Read the model definition and answer for the solid it produces. Units are mm, in the model's axes. A direction names the side the tool comes from. Coordinates: 2 decimals unless noted, no trailing zeros. Loops run counter-clockwise (first coordinate to the right, second up) from the corner with the lowest first, then second, coordinate; pieces in that order, holes last. Notation, with made-up numbers: (75, 17.5) -> (85, 17.5) arc R20 ccw to (85, 46.5) -> close; hole circle Ø5 at (-13.5, -26). An arc over 180 degrees is marked (long way). Answer as a JSON object with one key per item and string values. Group by question number.
1) Section C-C, the plane x = -3.5 is taken. Give the vertices of the cut face in (y, z), plus the area to 3 significant figures.
2) Section D-D, the plane y = -82.5 is taken. Give the vertices of the cut face in (x, z), plus the area to 3 significant figures.
3) Section B-B, the plane z = 4.4 is taken. Count the separate pieces of the cut face and the enclosed holes in it, plus the area to 3 significant figures.
4) A flat-ended cylindrical pin translates along its axis: P1, Ø3, axis at x = -23.5, z = 3.5, coming from the -Y side. Find the tip coordinate at first contact, or state that the pin passes through.
5) Consider probe 1 along Y at (x, z) = (-23.75, 2); probe 2 along X at (y, z) = (-16, 0.45); probe 3 along Y at (x, z) = (23.75, 1.7). Determine where each line is inside the solid, lowest interval first. Write a range as [from, to].
6) Section A-A, the plane y = 2.58 is taken. Give the vertices of the cut face in (x, z).
7) Determine the mould class of faces 1 (the face through (-49.907, 6.677, 2.839)), 2 (the face through (-6, 12.5, 3)), 3 (the face through (-53.41, -49.93, 2.76)) for opening direction X: released by +X, released by -X, zero draft, split by the parting line, or undercut.
8) Which of the six approach directions +Z, -Z, +X, -X, +Y, -Y give full straight-line access (tool end or side, diameter ignored) to faces 4 (the face through (-20, -3, 3)), 5 (the face through (-63.37, -66.79, 2.84)), 6 (the face through (-23, -12.5, 3))?
from build123d import *

# Parameters (mm, degrees)
BOSS_EXTRU_1_DEPTH      = 5.6
ENL_V_MAT_EXTRU_1_REACH = 135.059
ESQUISSE2_W             = 40
ESQUISSE2_H             = 20
ENL_V_MAT_EXTRU_2_REACH = 135.059
ESQUISSE3_R             = 1.45
CONG_2_R                = 12.5
CONG_3_R                = 10
CONG_4_R                = 30
CONG_5_R                = 30
ENL_V_MAT_EXTRU_3_REACH = 135.059
CONG_6_R                = 2
ENL_V_MAT_EXTRU_4_REACH = 135.059
ESQUISSE5_R             = 1.15


# Some blends are built 0.0001 mm under size
with BuildPart() as part:
    # Esquisse1 → Boss.-Extru.1 (new body)
    with BuildSketch(Plane.XY):
        with BuildLine():
            Line((-32.5, 12.5), (-52.5, 12.5))
            ThreePointArc((-52.5, 12.5), (-69.287355537, -46.339080558), (-67.5, -107.5))
            ThreePointArc((-67.5, -107.5), (-62.5, -112.5), (-57.5, -107.5))
            ThreePointArc((-57.5, -107.5), (-48.914858734, -58.969774017), (-32.5, -12.5))
            Line((-32.5, -12.5), (32.5, -12.5))
            Line((32.5, -12.5), (32.5, 12.5))
            Line((32.5, 12.5), (-32.5, 12.5))
        make_face()
    extrude(amount=BOSS_EXTRU_1_DEPTH)

    # Esquisse2 → Enlèv. mat.-Extru.1 (cut, up to next)
    with BuildSketch(Plane.XY.offset(5.6), mode=Mode.PRIVATE) as enl_v_mat_extru_1_sk1:
        with Locations((0, -2.5)):
            Rectangle(ESQUISSE2_W, ESQUISSE2_H)
    enl_v_mat_extru_1_tool1 = extrude(enl_v_mat_extru_1_sk1.sketch, amount=-ENL_V_MAT_EXTRU_1_REACH, mode=Mode.PRIVATE) & part.part
    add(enl_v_mat_extru_1_tool1.solids().sort_by_distance((0, -2.5, 5.6))[0], mode=Mode.SUBTRACT)

    # Esquisse3 → Enlèv. mat.-Extru.2 (cut, up to next)
    with BuildSketch(Plane.XY.offset(5.6), mode=Mode.PRIVATE) as enl_v_mat_extru_2_sk1:
        with Locations((-23.75, -7.58)):
            Circle(ESQUISSE3_R)
    enl_v_mat_extru_2_tool1 = extrude(enl_v_mat_extru_2_sk1.sketch, amount=-ENL_V_MAT_EXTRU_2_REACH, mode=Mode.PRIVATE) & part.part
    # Esquisse3 → Enlèv. mat.-Extru.2 (cut, up to next)
    with BuildSketch(Plane.XY.offset(5.6), mode=Mode.PRIVATE) as enl_v_mat_extru_2_sk2:
        with Locations((23.75, -7.58)):
            Circle(ESQUISSE3_R)
    enl_v_mat_extru_2_tool2 = extrude(enl_v_mat_extru_2_sk2.sketch, amount=-ENL_V_MAT_EXTRU_2_REACH, mode=Mode.PRIVATE) & part.part
    # Esquisse3 → Enlèv. mat.-Extru.2 (cut, up to next)
    with BuildSketch(Plane.XY.offset(5.6), mode=Mode.PRIVATE) as enl_v_mat_extru_2_sk3:
        with Locations((23.75, 2.58)):
            Circle(ESQUISSE3_R)
    enl_v_mat_extru_2_tool3 = extrude(enl_v_mat_extru_2_sk3.sketch, amount=-ENL_V_MAT_EXTRU_2_REACH, mode=Mode.PRIVATE) & part.part
    # Esquisse3 → Enlèv. mat.-Extru.2 (cut, up to next)
    with BuildSketch(Plane.XY.offset(5.6), mode=Mode.PRIVATE) as enl_v_mat_extru_2_sk4:
        with Locations((-23.75, 2.58)):
            Circle(ESQUISSE3_R)
    enl_v_mat_extru_2_tool4 = extrude(enl_v_mat_extru_2_sk4.sketch, amount=-ENL_V_MAT_EXTRU_2_REACH, mode=Mode.PRIVATE) & part.part
    add(enl_v_mat_extru_2_tool1.solids().sort_by_distance((-23.75, -7.58, 5.6))[0], mode=Mode.SUBTRACT)
    add(enl_v_mat_extru_2_tool2.solids().sort_by_distance((23.75, -7.58, 5.6))[0], mode=Mode.SUBTRACT)
    add(enl_v_mat_extru_2_tool3.solids().sort_by_distance((23.75, 2.58, 5.6))[0], mode=Mode.SUBTRACT)
    add(enl_v_mat_extru_2_tool4.solids().sort_by_distance((-23.75, 2.58, 5.6))[0], mode=Mode.SUBTRACT)

    # Congé2
    cong_2_edges = [part.edges().sort_by_distance(p)[0] for p in [
        (32.5, -12.5, 2.8),
        (32.5, 12.5, 2.8),
    ]]
    fillet(cong_2_edges, radius=CONG_2_R - 0.0001)  # a hair under: the kernel refuses the full size

    # Congé3
    cong_3_edges = [part.edges().sort_by_distance(p)[0] for p in [
        (-32.5, -12.5, 2.8),
    ]]
    fillet(cong_3_edges, radius=CONG_3_R)

    # Congé4
    cong_4_edges = [part.edges().sort_by_distance(p)[0] for p in [
        (-52.5, 12.5, 2.8),
    ]]
    fillet(cong_4_edges, radius=CONG_4_R)

    # Congé5
    # the kernel refuses this fillet: 30 mm, written as the material it adds along each edge
    with BuildSketch(Plane(origin=(-57.5, -107.5, 0), x_dir=(-0.029294676062998543, -0.9995708188789647, 0), z_dir=(0, 0, 1))) as cong_5_piece_1:
        with BuildLine():
            CenterArc((1.171787043, 29.987124566), CONG_5_R, 266.202223448, 2.119075089)
            ThreePointArc((-0.815268333, 0.053003384), (-0.407652209, 0.026224165), (0, 0))
            ThreePointArc((0, 0), (0.14647338, 0.002145906), (0.292946761, 0))
        make_face()
    extrude(amount=5.6)

    # Esquisse4 → Enlèv. mat.-Extru.3 (cut, up to next)
    with BuildSketch(Plane.XY.offset(5.6), mode=Mode.PRIVATE) as enl_v_mat_extru_3_sk1:
        Polygon((-35.530484253, -6.741676359), (-42.974151572, -20.332321303), (-48.555833289, 0.989708193), align=None)
    enl_v_mat_extru_3_tool1 = extrude(enl_v_mat_extru_3_sk1.sketch, amount=-ENL_V_MAT_EXTRU_3_REACH, mode=Mode.PRIVATE) & part.part
    # Esquisse4 → Enlèv. mat.-Extru.3 (cut, up to next)
    with BuildSketch(Plane.XY.offset(5.6), mode=Mode.PRIVATE) as enl_v_mat_extru_3_sk2:
        Polygon((-52.982896502, -3.816878406), (-45.919055028, -30.800759586), (-62.900626013, -49.913479621), align=None)
    enl_v_mat_extru_3_tool2 = extrude(enl_v_mat_extru_3_sk2.sketch, amount=-ENL_V_MAT_EXTRU_3_REACH, mode=Mode.PRIVATE) & part.part
    # Esquisse4 → Enlèv. mat.-Extru.3 (cut, up to next)
    with BuildSketch(Plane.XY.offset(5.6), mode=Mode.PRIVATE) as enl_v_mat_extru_3_sk3:
        Polygon((-49.898192375, -43.559912364), (-63.702500518, -59.0966302), (-62.552958266, -85.696486809), align=None)
    enl_v_mat_extru_3_tool3 = extrude(enl_v_mat_extru_3_sk3.sketch, amount=-ENL_V_MAT_EXTRU_3_REACH, mode=Mode.PRIVATE) & part.part
    add(enl_v_mat_extru_3_tool1.solids().sort_by_distance((-42.35349, -8.694763, 5.6))[0], mode=Mode.SUBTRACT)
    add(enl_v_mat_extru_3_tool2.solids().sort_by_distance((-53.934193, -28.177039, 5.6))[0], mode=Mode.SUBTRACT)
    add(enl_v_mat_extru_3_tool3.solids().sort_by_distance((-58.717884, -62.784343, 5.6))[0], mode=Mode.SUBTRACT)

    # Congé6
    cong_6_edges = [part.edges().sort_by_distance(p)[0] for p in [
        (-48.555833289, 0.989708193, 2.8),
        (-35.530484253, -6.741676359, 2.8),
        (-42.974151572, -20.332321303, 2.8),
        (-62.900626013, -49.913479621, 2.8),
        (-52.982896502, -3.816878406, 2.8),
        (-45.919055028, -30.800759586, 2.8),
        (-49.898192375, -43.559912364, 2.8),
        (-62.552958266, -85.696486809, 2.8),
        (-63.702500518, -59.0966302, 2.8),
    ]]
    fillet(cong_6_edges, radius=CONG_6_R)

    # Esquisse5 → Enlèv. mat.-Extru.4 (cut, up to next)
    with BuildSketch(Plane.XY.offset(5.6), mode=Mode.PRIVATE) as enl_v_mat_extru_4_sk1:
        with Locations((15, 9.91)):
            Circle(ESQUISSE5_R)
    enl_v_mat_extru_4_tool1 = extrude(enl_v_mat_extru_4_sk1.sketch, amount=-ENL_V_MAT_EXTRU_4_REACH, mode=Mode.PRIVATE) & part.part
    # Esquisse5 → Enlèv. mat.-Extru.4 (cut, up to next)
    with BuildSketch(Plane.XY.offset(5.6), mode=Mode.PRIVATE) as enl_v_mat_extru_4_sk2:
        with Locations((5, 9.91)):
            Circle(ESQUISSE5_R)
    enl_v_mat_extru_4_tool2 = extrude(enl_v_mat_extru_4_sk2.sketch, amount=-ENL_V_MAT_EXTRU_4_REACH, mode=Mode.PRIVATE) & part.part
    add(enl_v_mat_extru_4_tool1.solids().sort_by_distance((15, 9.91, 5.6))[0], mode=Mode.SUBTRACT)
    add(enl_v_mat_extru_4_tool2.solids().sort_by_distance((5, 9.91, 5.6))[0], mode=Mode.SUBTRACT)


solid = part.part
Determined:
{
 "1": {"outline": "(7.5, 0) -> (12.5, 0) -> (12.5, 5.6) -> (7.5, 5.6) -> close", "area": "28.0 mm²"},
 "2": {"outline": "(-70.51, 0) -> (-54.11, 0) -> (-54.11, 5.6) -> (-70.51, 5.6) -> close", "area": "91.9 mm²"},
 "3": {"separate pieces": "1", "enclosed holes": "9", "area": "2,750 mm²"},
 "4": {"P1": "y = -12.5"},
 "5": {"probe 1": "[-12.5, -9.03], [-6.13, 1.13], [4.03, 12.5]", "probe 2": "[-63.08, -55.6], [-49.79, -44.02], [-40.6, -33.55]", "probe 3": "[-11.92, -9.03], [-6.13, 1.13], [4.03, 11.92]"},
 "6": {"outline": "(-54.43, 0) -> (-25.2, 0) -> (-25.2, 5.6) -> (-54.43, 5.6) -> close; (-22.3, 0) -> (-20, 0) -> (-20, 5.6) -> (-22.3, 5.6) -> close; (20, 0) -> (22.3, 0) -> (22.3, 5.6) -> (20, 5.6) -> close; (25.2, 0) -> (32.23, 0) -> (32.23, 5.6) -> (25.2, 5.6) -> close"},
 "7": {"face 1": "released by -X", "face 2": "zero draft", "face 3": "undercut"},
 "8": {"face 4": "+Z, -Z, -Y", "face 5": "+Z, -Z", "face 6": "+Z, -Z, +X, -Y"}
}
